from build123d import *

# Parameters (mm, degrees)
F4_R     = 5
F5_DEPTH = 2.5


with BuildPart() as f2:
    # F2: sweep along a path in F0
    with BuildLine(Plane.XZ) as f2_path:
        Line((0, 60), (-90, 60))
        ThreePointArc((-90, 60), (-97.0710678119, 57.0710678119), (-100, 50))
        Line((-100, 50), (-100, 0))
    # F1 (on Right) → F2 (sweep)
    with BuildSketch(Plane.YZ):
        with BuildLine():
            Line((10, 95), (10, 100))
            Line((10, 100), (-10, 100))
            Line((-10, 100), (-10, 95))
            Line((-10, 95), (-5.5, 95))
            ThreePointArc((-5.5, 95), (-3.3786796564, 94.1213203436), (-2.5, 92))
            Line((-2.5, 92), (-2.5, 68))
            ThreePointArc((-2.5, 68), (-3.3786796564, 65.8786796564), (-5.5, 65))
            Line((-5.5, 65), (-10, 65))
            Line((-10, 65), (-10, 60))
            Line((-10, 60), (0, 60))
            Line((0, 60), (10, 60))
            Line((10, 60), (10, 65))
            Line((10, 65), (5.5, 65))
            ThreePointArc((5.5, 65), (3.3786796564, 65.8786796564), (2.5, 68))
            Line((2.5, 68), (2.5, 92))
            ThreePointArc((2.5, 92), (3.3786796564, 94.1213203436), (5.5, 95))
            Line((5.5, 95), (10, 95))
        make_face()
    sweep(path=f2_path.line)

    # F3: F2 across plane


with BuildPart() as f2_1:
    add(f2.part)
    add(f2.part.mirror(Plane.XY))

    # F4 (on Front) → F5 (join, symmetric)
    with BuildSketch(Plane.XZ):
        with BuildLine():
            Line((0, 100), (0, 130))
            ThreePointArc((0, 130), (-13.3277028936, 148.8541892248), (-35.5480451324, 142.5800752207))
            Line((-35.5480451324, 142.5800752207), (-70, 100))
            Line((-70, 100), (0, 100))
        make_face()
        with Locations((-20, 130)):
            Circle(F4_R, mode=Mode.SUBTRACT)
        with BuildLine():
            Line((0, -100), (-70, -100))
            Line((-70, -100), (-35.5480451324, -142.5800752207))
            ThreePointArc((-35.5480451324, -142.5800752207), (-13.3277028936, -148.8541892248), (0, -130))
            Line((0, -130), (0, -100))
        make_face()
        with Locations((-20, -130)):
            Circle(F4_R, mode=Mode.SUBTRACT)
    extrude(amount=F5_DEPTH, both=True)


solid = f2_1.part
The model under review builds one solid part; all positions refer to its coordinate system, in mm. A direction names the side the tool comes from. Give positions to 0.01 mm unless a question says otherwise; leave off trailing zeros. Order: outer loops, then holes, each group sorted by start corner. A loop starts at its lowest first (then second) coordinate and runs counter-clockwise, first axis right, second up. Notation, with made-up numbers: M 82.5,-23.75 L 104.5,-23.75 A6 ccw 104.5,-13.75 Z; hole C 8.25,-15.75 d3. An arc over 180 degrees is marked long. Answer in a Markdown table with one row per item. Add a question column.
1. Mouldability with a two-part tool opening along X and no side actions: class faces 1 (the flat face through (-28, -2.5, 120)), 2 (the flat face through (-111, -2.5, -1)), 3 (the flat face through (-52.53, 0.04, 121.59)) as released by +X, released by -X, zero draft, split by the parting line, or undercut.
2. To check wall thickness, follow line 1 along Z through (x, y) = (-20, 1.15); line 2 along Z through (x, y) = (-44.5, -8); line 3 along X through (y, z) = (-8, 3.5). State the ranges of each line that lie inside material, in increasing order.
3. Add section A-A on z = -44.5. State the section outline as (x, y) points, plus the area to 3 significant figures.
4. Machinability: for faces 4 (the flat face through (-28, 2.5, 120)), 5 (the cylindrical face through (-100.49, -7.78, -60.72)), 6 (the cylindrical face through (-121.468, 7.781, 82.168)), 7 (the flat face through (-103, 10, 0)), 8 (the cylindrical face through (-96.99, 0.14, 57.15)), which of the approach directions +Z, -Z, +X, -X, +Y, -Y give a long, thin tool a straight path to every point of the face, cutting with its end or side? Answer none if there is none.
5. Add section B-B on x = -20. Count the separate pieces of the cut face and the enclosed holes in it, plus the area to 3 significant figures.
6. For pin 1 Ø5 at (x, y) = (-63.5, -8.5) entering from +Z; pin 2 Ø8 at (x, z) = (-20, -130) entering from -Y; pin 3 Ø8 at (x, y) = (-123, -0.5) entering from +Z; pin 4 Ø10 at (x, y) = (-104.5, -0.5) entering from +Z, all flat-tipped, find the tip position at first contact; note any pin that passes through.
The answers:
| question | item | result |
|---|---|---|
| 1 | face 1 | zero draft |
| 1 | face 2 | undercut |
| 1 | face 3 | released by -X |
| 2 | line 1 | -150 to -135, -125 to -60, 60 to 125, 135 to 150 |
| 2 | line 2 | -100 to -95, -65 to -60, 60 to 65, 95 to 100 |
| 2 | line 3 | -140 to -135, -105 to -100 |
| 3 | outline | M -140,-10 L -135,-10 L -135,-5.5 A3 cw -132,-2.5 L -108,-2.5 A3 cw -105,-5.5 L -105,-10 L -100,-10 L -100,10 L -105,10 L -105,5.5 A3 cw -108,2.5 L -132,2.5 A3 cw -135,5.5 L -135,10 L -140,10 Z |
| 3 | area | 358 mm2 |
| 4 | face 4 | +Z, +X, -X, +Y |
| 4 | face 5 | -Y |
| 4 | face 6 | +Y |
| 4 | face 7 | +Z, -Z, +X, -X, +Y |
| 4 | face 8 | +X, +Y, -Y |
| 5 | separate pieces | 4 |
| 5 | enclosed holes | 0 |
| 5 | area | 1,120 mm2 |
| 6 | pin 1 | z = 100 |
| 6 | pin 2 | through |
| 6 | pin 3 | z = 90.73 |
| 6 | pin 4 | z = 99.09 |
